Read the model definition and answer for the solid it produces. Units are mm, in the model's axes. A direction names the side the tool comes from. Coordinates: 2 decimals unless noted, no trailing zeros. Loops run counter-clockwise (first coordinate to the right, second up) from the corner with the lowest first, then second, coordinate; pieces in that order, holes last.
Q1. Section C-C (z = 13.75) is taken. Give the vertices of the cut face in (x, y), then the cut area to 3 significant figures.
Q2. Section B-B (x = 0) is taken. Give the vertices of the cut face in (y, z).
Q3. Straight lines are drawn through the part: line 1 (X direction, y = 0.25, z = 13); line 2 (Y direction, x = 0, z = 2.5); line 3 (Z direction, x = 12, y = 0.5). For each, find the intervals that lie inside material, in ascending order.
Q4. Which of the six approach directions +Z, -Z, +X, -X, +Y, -Y give full straight-line access (tool end or side, diameter ignored) to faces 1 (the face through (0, 5, 12)), 2 (the face through (-17, 0, 15)), 3 (the face through (2, -2, 7))?
Q5. Section A-A (y = 0) is taken. Give the vertices of the cut face in (x, z), then the cut area to 3 significant figures.
Q6. Section D-D (z = 9.75) is taken. Give the vertices of the cut face in (x, y), then the cut area to 3 significant figures.
Q7. A flat-ended cylindrical pin translates along its axis: P1, Ø5, axis at x = 3.5, y = 4, coming from the +Z side. Find the tip coordinate at first contact, or state that the pin passes through.
Q8. The mould has two halves that part along Y. Classify faces 4 (the face through (0, 10, 6)), 5 (the face through (-0.54, -2.44, 3.45)), 6 (the face through (-0.59, 4.46, 9.54)), 7 (the face through (-13.5, 0, 14)): pulls with the +Y half, pulls with the -Y half, needs draft (parallel to the pull), parting line crosses it, or undercut.
from build123d import *

# Parameters (mm, degrees)
F0_W     = 40
F0_H     = 20
F0_R     = 2.5
F1_DEPTH = 15
F2_W     = 27
F2_H     = 20
F2_R     = 2.5
F3_DEPTH = 3
F4_R     = 4.5
F5_DEPTH = 5


with BuildPart() as f1:
    # F0 (on Top) → F1 (new body)
    with BuildSketch(Plane.XY):
        Rectangle(F0_W, F0_H)
        Circle(F0_R, mode=Mode.SUBTRACT)
    extrude(amount=F1_DEPTH)

    # F2 (on face) → F3 (cut)
    with BuildSketch(Plane.XY.offset(15)):
        Rectangle(F2_W, F2_H)
        Circle(F2_R, mode=Mode.SUBTRACT)
    extrude(amount=-F3_DEPTH, mode=Mode.SUBTRACT)

    # F4 (on face) → F5 (cut)
    with BuildSketch(Plane.XY.offset(12)):
        Circle(F4_R)
    extrude(amount=-F5_DEPTH, mode=Mode.SUBTRACT)


solid = f1.part
Numbers:
1. outline: (-20, -10) - (-13.5, -10) - (-13.5, 10) - (-20, 10) - close; (13.5, -10) - (20, -10) - (20, 10) - (13.5, 10) - close
1. area: 260 mm2
2. outline: (-10, 0) - (-2.5, 0) - (-2.5, 7) - (-4.5, 7) - (-4.5, 12) - (-10, 12) - close; (2.5, 0) - (10, 0) - (10, 12) - (4.5, 12) - (4.5, 7) - (2.5, 7) - close
3. line 1: x = -20 to -13.5, 13.5 to 20
3. line 2: y = -10 to -2.5, 2.5 to 10
3. line 3: z = 0 to 12
4. face 1: +Z, +Y, -Y
4. face 2: +Z, +X, -X, +Y, -Y
4. face 3: +Z
5. outline: (-20, 0) - (-2.5, 0) - (-2.5, 7) - (-4.5, 7) - (-4.5, 12) - (-13.5, 12) - (-13.5, 15) - (-20, 15) - close; (2.5, 0) - (20, 0) - (20, 15) - (13.5, 15) - (13.5, 12) - (4.5, 12) - (4.5, 7) - (2.5, 7) - close
5. area: 439 mm2
6. outline: (-20, -10) - (20, -10) - (20, 10) - (-20, 10) - close; hole circle Ø9 at (0, 0)
6. area: 736 mm2
7. P1: stops at z = 12
8. face 4: pulls with the +Y half
8. face 5: undercut
8. face 6: undercut
8. face 7: needs draft
